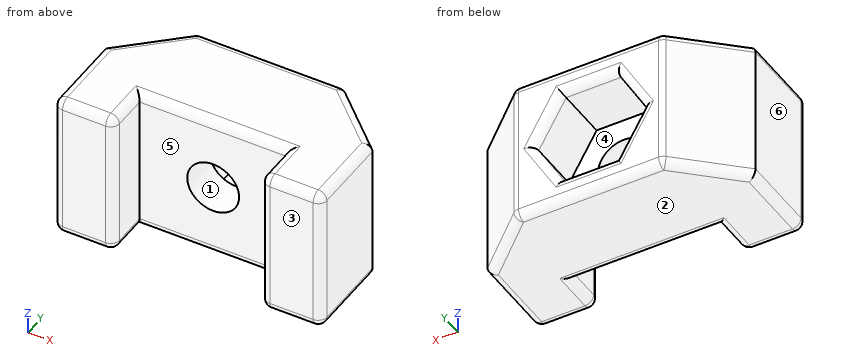
```python
from build123d import *

# Parameters (mm, degrees)
BOSS_EXTRU_1_DEPTH      = 17
ENL_V_MAT_EXTRU_1_DEPTH = 7
ESQUISSE3_R             = 3
ENL_V_MAT_EXTRU_2_DEPTH = 5
CONG_1_R                = 1


with BuildPart() as part:
    # Esquisse1 → Boss.-Extru.1 (new body)
    with BuildSketch(Plane.XY):
        Polygon((-3, 1.840029022), (3, 1.840029022), (8.5, 1.840029022), (8.5, -3.159970978), (15.5, -3.159970978), (15.5, 6.840029022), (8.5, 13.340029022), (-8.5, 13.340029022), (-15.5, 6.840029022), (-15.5, -3.159970978), (-8.5, -3.159970978), (-8.5, 1.840029022), align=None)
    extrude(amount=BOSS_EXTRU_1_DEPTH)

    # Esquisse2 → Enlèv. mat.-Extru.1 (cut)
    with BuildSketch(Plane(origin=(0, 13.340029022, 0), x_dir=(1, 0, 0), z_dir=(0, 1, 0))):
        Polygon((6.350852961, -8.5), (3.175426481, -3), (-3.175426481, -3), (-6.350852961, -8.5), (-3.175426481, -14), (3.175426481, -14), align=None)
    extrude(amount=-ENL_V_MAT_EXTRU_1_DEPTH, mode=Mode.SUBTRACT)

    # Esquisse3 → Enlèv. mat.-Extru.2 (cut)
    with BuildSketch(Plane(origin=(0, 6.340029022, 0), x_dir=(1, 0, 0), z_dir=(0, 1, 0))):
        with Locations(Location((0, -8.5, 0), (0, 0, 270))):
            Circle(ESQUISSE3_R)
    extrude(amount=-ENL_V_MAT_EXTRU_2_DEPTH, mode=Mode.SUBTRACT)

    # Congé1
    cong_1_edges = [part.edges().sort_by_distance(p)[0] for p in [
        (12, -3.159970978, 17),
        (0, 1.840029022, 0),
        (-8.5, -0.659970978, 0),
        (-12, -3.159970978, 0),
        (-15.5, 1.840029022, 0),
        (-12, 10.090029022, 0),
        (15.5, 1.840029022, 17),
        (0, 13.340029022, 0),
        (12, 10.090029022, 0),
        (15.5, 1.840029022, 0),
        (12, -3.159970978, 0),
        (8.5, -0.659970978, 0),
        (12, 10.090029022, 17),
        (0, 13.340029022, 17),
        (-8.5, -3.159970978, 8.5),
        (-15.5, -3.159970978, 8.5),
        (-8.5, 13.340029022, 8.5),
        (8.5, 13.340029022, 8.5),
        (15.5, -3.159970978, 8.5),
        (8.5, -3.159970978, 8.5),
        (-12, 10.090029022, 17),
        (-15.5, 1.840029022, 17),
        (-12, -3.159970978, 17),
        (-8.5, -0.659970978, 17),
        (0, 1.840029022, 17),
        (4.763139721, 13.340029022, 11.25),
        (4.763139721, 13.340029022, 5.75),
        (0, 13.340029022, 3),
        (-4.763139721, 13.340029022, 5.75),
        (-4.763139721, 13.340029022, 11.25),
        (0, 13.340029022, 14),
        (8.5, -0.659970978, 17),
    ]]
    fillet(cong_1_edges, radius=CONG_1_R)


solid = part.part
```
Model file for the job. Use its own axes, mm. Face numbers are marked on the shaded views. A direction names the side the tool comes from. Coordinates: 2 decimals unless noted, no trailing zeros. Order: outer loops, then holes, each group sorted by start corner. A loop starts at its lowest first (then second) coordinate and runs counter-clockwise, first axis right, second up. Notation, with made-up numbers: (3, -14.5) - (32, -14.5) arc R18 ccw to (32, -6.5) - close; hole circle Ø11 at (-18, 21). An arc over 180 degrees is marked (long way). Return JSON: item names as keys, results as strings. Group by question number.
1) Tool access for the marked faces 4, 5 and 6: list every direction of +Z, -Z, +X, -X, +Y, -Y with a clear straight run to the whole face (end or side of a thin tool).
2) Mould opens along Z. For the marked faces 1, 2 and 3 say: released by +Z, released by -Z, zero draft, split by the parting line, or undercut.
3) Flat gauge pins, fed straight in: P1, Ø3, axis at x = -2.5, z = 6.5, coming from the +Y side; P2, Ø8, axis at x = 0, z = 8.5, coming from the -Y side. Where does each tip first touch, or does it go through?
4) Probe line 1 (X direction, y = 5.1, z = 8.5); line 2 (Y direction, x = 3.5, z = 2); line 3 (Y direction, x = 1, z = 12.5). List the from-to ranges inside material, lowest first. Write a range as from..to.
5) Saw through at B-B, the plane y = 5.75. Write the cut outline in (x, z), plus the area to 3 significant figures.
6) Saw through at C-C, the plane y = 2.5. Write the cut outline in (x, z).
7) Saw through at A-A, the plane x = 0. Write the cut outline in (y, z).
Values found:
{
 "1": {"face 4": "+Y", "face 5": "+Z, -Z, -Y", "face 6": "+Z, -Z, -X, +Y, -Y"},
 "2": {"face 1": "undercut", "face 2": "released by -Z", "face 3": "zero draft"},
 "3": {"P1": "stops at y = 6.34", "P2": "stops at y = 1.84"},
 "4": {"line 1": "x = -15.5..-3, 3..15.5", "line 2": "y = 1.84..13.34", "line 3": "y = 1.84..6.34"},
 "5": {"outline": "(-15.5, 1) arc R1 ccw to (-14.5, 0) - (14.5, 0) arc R1 ccw to (15.5, 1) - (15.5, 16) arc R1 ccw to (14.5, 17) - (-14.5, 17) arc R1 ccw to (-15.5, 16) - close; hole circle Ø6 at (0, 8.5)", "area": "498 mm²"},
 "6": {"outline": "(-15.5, 1) arc R1 ccw to (-14.5, 0) - (-9.5, 0) arc R1 ccw to (-9.16, 0.06) - (9.16, 0.06) arc R1 ccw to (9.5, 0) - (14.5, 0) arc R1 ccw to (15.5, 1) - (15.5, 16) arc R1 ccw to (14.5, 17) - (9.5, 17) arc R1 ccw to (9.16, 16.94) - (-9.16, 16.94) arc R1 ccw to (-9.5, 17) - (-14.5, 17) arc R1 ccw to (-15.5, 16) - close; hole circle Ø6 at (0, 8.5)"},
 "7": {"outline": "(1.84, 1) arc R1 ccw to (2.84, 0) - (12.34, 0) arc R1 ccw to (13.34, 1) - (13.34, 2) arc R1 ccw to (12.34, 3) - (6.34, 3) - (6.34, 5.5) - (1.84, 5.5) - close; (1.84, 11.5) - (6.34, 11.5) - (6.34, 14) - (12.34, 14) arc R1 ccw to (13.34, 15) - (13.34, 16) arc R1 ccw to (12.34, 17) - (2.84, 17) arc R1 ccw to (1.84, 16) - close"}
}
